```python
from build123d import *

# Parameters (mm, degrees)
F1_DEPTH = 88
F2_R     = 2
F3_DEPTH = 8.1


with BuildPart() as f1:
    # F0 (on Front) → F1 (new body)
    with BuildSketch(Plane.XZ):
        Polygon((-1.34, 4), (-4, 4), (-4, -4), (4, -4), (4, 4), (1.34, 4), (1.34, -2.75), (-1.34, -2.75), align=None)
    extrude(amount=F1_DEPTH)

    # F2 (on face) → F3 (cut)
    with BuildSketch(Plane.YZ.offset(4)):
        with Locations((-84, 0)):
            Circle(F2_R)
        with Locations((-68, 0)):
            Circle(F2_R)
        with Locations((-52, 0)):
            Circle(F2_R)
        with Locations((-36, 0)):
            Circle(F2_R)
        with Locations((-20, 0)):
            Circle(F2_R)
        with Locations((-6, 0)):
            Circle(F2_R)
    extrude(amount=-F3_DEPTH, mode=Mode.SUBTRACT)


solid = f1.part
```
The model under review builds one solid part; all positions refer to its coordinate system, in mm. A direction names the side the tool comes from. Round coordinates to 2 decimals unless told otherwise and drop trailing zeros. Loops run counter-clockwise (first coordinate to the right, second up) from the corner with the lowest first, then second, coordinate; pieces in that order, holes last.
Item 1: Take a section at A-A (y = -6). Write out the cut boundary in (x, z).
Determined:
outline: (-4, -4) - (4, -4) - (4, -2) - (1.34, -2) - (1.34, -2.75) - (-1.34, -2.75) - (-1.34, -2) - (-4, -2) - close; (-4, 2) - (-1.34, 2) - (-1.34, 4) - (-4, 4) - close; (1.34, 2) - (4, 2) - (4, 4) - (1.34, 4) - close
Item 2: Take a section at C-C (y = -57). Write out the cut boundary in (x, z), then the cut area to 3 significant figures.
Determined:
outline: (-4, -4) - (4, -4) - (4, 4) - (1.34, 4) - (1.34, -2.75) - (-1.34, -2.75) - (-1.34, 4) - (-4, 4) - close
area: 45.9 mm2
Item 3: Take a section at B-B (x = 2.75). Write out the cut boundary in (y, z).
Determined:
outline: (-88, -4) - (0, -4) - (0, 4) - (-88, 4) - close; hole circle Ø4 at (-84, 0); hole circle Ø4 at (-68, 0); hole circle Ø4 at (-52, 0); hole circle Ø4 at (-36, 0); hole circle Ø4 at (-20, 0); hole circle Ø4 at (-6, 0)
Item 4: For line 1 (X direction, y = -65, z = -1.25); line 2 (Z direction, x = 2.7, y = -84); line 3 (Z direction, x = -0.5, y = -75), list the stretches that pass through material, from the lowest coordinate up.
Determined:
line 1: x = -4 to -1.34, 1.34 to 4
line 2: z = -4 to -2, 2 to 4
line 3: z = -4 to -2.75
Item 5: For faces 1 (the face through (-3, -38, 0)), 2 (the face through (1.34, -43, 1)), list the 3-axis set-ups (+Z, -Z, +X, -X, +Y, -Y) from which the entire face can be reached by the end or side of a thin tool; tool diameter is ignored.
Determined:
face 1: +X, -X
face 2: +Z, +Y, -Y
Item 6: Mouldability with a two-part tool opening along Y and no side actions: class faces 3 (the face through (0, -43, -2.75)), 4 (the face through (3, -38, 0)), 5 (the face through (-2, 0, 0)) as released by +Y, released by -Y, zero draft, split by the parting line, or undercut.
Determined:
face 3: zero draft
face 4: undercut
face 5: released by +Y
Item 7: Take a section at D-D (z = 1.25). Give the number of separate pieces and of enclosed holes in the cut face, then the cut area to 3 significant figures.
Determined:
separate pieces: 14
enclosed holes: 0
area: 368 mm2
Item 8: Clearance check with a flat-ended pin moving along its axis: pin 1 Ø1.3 at (x, y) = (0, -52) entering from +Z. State where the tip first meets the part, or that it passes through.
Determined:
pin 1: stops at z = -2.75
